Here's how the part is built. I have some questions about the finished solid (model axes, mm). Give positions to 0.01 mm unless a question says otherwise; leave off trailing zeros. Order: outer loops, then holes, each group sorted by start corner. A loop starts at its lowest first (then second) coordinate and runs counter-clockwise, first axis right, second up. Notation, with made-up numbers: (1, 55) - (27, 55) arc R22 cw to (27, 79) - close; hole circle Ø8 at (55.5, 3.5). An arc over 180 degrees is marked (long way). One line per question, with ' | ' between items.
from build123d import *

# Parameters (mm, degrees)
BOSS_EXTRUDE1_DEPTH    = 6.35
CUT_EXTRUDE1_DEPTH     = 7.35
F_10_CLEARANCE_HOLE1_D = 5.1054


with BuildPart() as part:
    # Sketch1 → Boss-Extrude1 (new body)
    with BuildSketch(Plane(origin=(0, 0, 0), x_dir=(0, 0, -1), z_dir=(1, 0, 0))):
        Polygon((257.81, 0), (-257.81, 0), (-95.25, 227.241295543), (95.25, 227.241295543), align=None)
    extrude(amount=BOSS_EXTRUDE1_DEPTH)

    # Sketch3 → Cut-Extrude1 (cut, through all)
    with BuildSketch(Plane(origin=(6.35, 0, 0), x_dir=(0, 0, -1), z_dir=(1, 0, 0))):
        Polygon((-47.089344398, 177.8), (47.089344398, 177.8), (101.6, 101.6), (101.6, 25.4), (-101.6, 25.4), (-101.6, 101.6), align=None)
    extrude(amount=-CUT_EXTRUDE1_DEPTH, mode=Mode.SUBTRACT)

    # #10 Clearance Hole1 (through all)
    with Locations(Plane(origin=(6.35, 0, 0), x_dir=(0, 0, -1), z_dir=(1, 0, 0))):
        with Locations((51.986786112, 187.325), (-51.986786112, 187.325), (111.125, 104.656174089), (111.125, 15.875), (-111.125, 15.875), (-111.125, 104.656174089), (0, 15.875)):
            Hole(F_10_CLEARANCE_HOLE1_D / 2)


solid = part.part
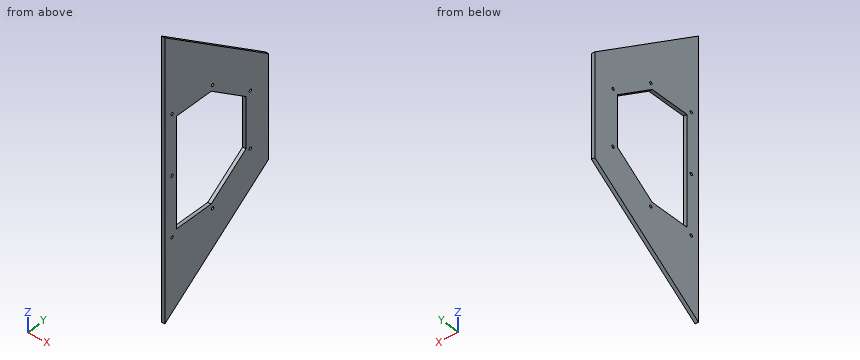
1) I want a section at B-B (x = 5). State how many separate pieces and enclosed holes the cut face has, plus the area to 3 significant figures.
Model answer:
separate pieces: 1 | enclosed holes: 8 | area: 53,300 mm2
2) I want a section at C-C (y = 54). List the corners of the cut face in (x, z) for me.
Model answer:
outline: (0, -219.18) - (6.35, -219.18) - (6.35, -101.6) - (0, -101.6) - close; (0, 101.6) - (6.35, 101.6) - (6.35, 219.18) - (0, 219.18) - close
3) I'm going to push flat-ended pins straight in: P1, Ø4.5, axis at y = 187.32, z = -51.99, coming from the -X side; P2, Ø1.9, axis at x = 3.5, y = 54, coming from the +Z side; P3, Ø3, axis at x = 4.5, y = 90.5, coming from the +Z side; P4, Ø3, axis at x = 2.5, y = 63, coming from the -Z side. Where does each tip first touch, or does it pass through?
Model answer:
P1: passes through | P2: stops at z = 219.86 | P3: stops at z = 194.14 | P4: stops at z = -213.82
4) I want a section at A-A (z = -15). List the corners of the cut face in (x, y) for me, plus the area to 3 significant figures.
Model answer:
outline: (0, 0) - (6.35, 0) - (6.35, 25.4) - (0, 25.4) - close; (0, 177.8) - (6.35, 177.8) - (6.35, 227.24) - (0, 227.24) - close | area: 475 mm2
5) Please list where these lines run through material, in increasing order: L1, parallel to Y at x = 2, z = 14; L2, parallel to Z at x = 2, y = 163; L3, parallel to Z at x = 2.75, y = 95.5.
Model answer:
L1: y = 0 to 25.4, 177.8 to 227.24 | L2: z = -141.21 to -57.68, 57.68 to 141.21 | L3: z = -189.49 to -101.6, 101.6 to 189.49
6) I want a section at D-D (z = -189.5). List the corners of the cut face in (x, y) for me.
Model answer:
outline: (0, 0) - (6.35, 0) - (6.35, 95.49) - (0, 95.49) - close
